Read the model definition and answer for the solid it produces. Units are mm, in the model's axes. A direction names the side the tool comes from. Coordinates: 2 decimals unless noted, no trailing zeros. Write each loop counter-clockwise with the first axis right and the second up, starting at its lowest first coordinate (ties: lowest second). Pieces come first, ordered by that corner, then holes. Notation, with made-up numbers: (50.5, 24.25) -> (62.5, 24.25) arc R16 cw to (62.5, 30.25) -> close; hole circle Ø6 at (63.5, 89). An arc over 180 degrees is marked (long way). Return JSON: item names as keys, results as strings.
Autodesk Inventor part; units mm, degrees
ref_plane "YZ Plane" through (0, 0, 0) normal (1, 0, 0) x (0, 1, 0)
ref_plane "XZ Plane" through (0, 0, 0) normal (0, 1, 0) x (-1, 0, 0)
ref_plane "XY Plane" through (0, 0, 0) normal (0, 0, 1) x (1, 0, 0)
sketch "스케치1" plane through (0, 0, 0) normal (0, 1, 0) x (-1, 0, 0)
  line L0 (24.089, 25.4241) -> (-27.911, 25.4241)
  line L1 (-27.911, 25.4241) -> (-27.911, -26.5759)
  line L2 (-27.911, -26.5759) -> (24.089, -26.5759)
  line L3 (24.089, -26.5759) -> (24.089, 25.4241)
  point P0 (0, 0)
  dimension "d0" = 52
  dimension "d1" = 52
extrude "돌출2" add sketch "스케치1" along normal blind 5
sketch "스케치2" plane through (0, 0, 0) normal (0, -1, 0) x (1, 0, 0)
  line L0 (27.911, 25.4241) -> (27.911, -26.5759)
  line L1 (-24.089, 25.4241) -> (27.911, 25.4241)
  line L2 (-24.089, -26.5759) -> (-24.089, 25.4241)
  line L3 (27.911, -26.5759) -> (-24.089, -26.5759)
  line L4 (-24.089, 25.4241) -> (-19.089, 25.4241)
  line L5 (-19.089, 25.4241) -> (-19.089, -26.5759)
  line L6 (-19.089, -26.5759) -> (-24.089, -26.5759)
  line L7 (-24.089, -26.5759) -> (-24.089, 25.4241)
  line L8 (27.911, 25.4241) -> (22.911, 25.4241)
  line L9 (22.911, 25.4241) -> (22.911, -26.5759)
  line L10 (22.911, -26.5759) -> (27.911, -26.5759)
  line L11 (27.911, -26.5759) -> (27.911, 25.4241)
  point P0 (0, 0)
  dimension "d8" = 5
  dimension "d9" = 5
extrude "돌출3" add sketch "스케치2" along normal blind 42 contours L0 L3 L9 L1 | L5 L3 L2 L1
sketch "스케치4" plane through (0, 5, 0) normal (0, 1, 0) x (1, 0, 0)
  line L0 (27.911, -25.4241) -> (27.911, 26.5759)
  line L1 (27.911, 26.5759) -> (-24.089, 26.5759)
  line L2 (-24.089, 26.5759) -> (-24.089, -25.4241)
  line L3 (-24.089, -25.4241) -> (27.911, -25.4241)
  line L4 (27.911, 26.5759) -> (38.911, 26.5759)
  line L5 (38.911, 26.5759) -> (38.911, -25.4241)
  line L6 (38.911, -25.4241) -> (27.911, -25.4241)
  line L7 (27.911, -25.4241) -> (27.911, 26.5759)
  line L8 (-24.089, 26.5759) -> (-36.089, 26.5759)
  line L9 (-36.089, 26.5759) -> (-36.089, -25.4241)
  line L10 (-36.089, -25.4241) -> (-24.089, -25.4241)
  line L11 (-24.089, -25.4241) -> (-24.089, 26.5759)
  line L12 (-24.089, 26.5759) -> (27.911, 26.5759)
  line L13 (27.911, 26.5759) -> (27.911, -25.4241)
  line L14 (27.911, -25.4241) -> (-24.089, -25.4241)
  line L15 (-24.089, -25.4241) -> (-24.089, 26.5759)
  line L16 (-24.089, -15.4219) -> (-4.089, -25.4241)
  point P0 (0, 0)
  point P1 (-24.089, -25.4241)
  dimension "d12" = 11
  dimension "d13" = 12
  dimension "d32" = 0
  dimension "d33" = 52
  dimension "d34" = 52
  dimension "d35" = 0
  dimension "d36" = 52
  dimension "d37" = 52
  dimension "d38" = 26.57
  dimension "d39" = 20
sketch "스케치8" plane through (27.911, -42, 25.4241) normal (1, 0, 0) x (0, 0, -1)
  line L0 (52, 0) -> (52, 47)
  line L1 (0, 47) -> (52, 47)
  line L2 (0, 47) -> (0, 0)
  line L3 (52, 0) -> (0, 0)
  circle A0 centre (26, 16.074) radius 4.5
  point P0 (25.4241, 42)
  point P1 (26, 0)
  dimension "d26" = 9
  dimension "d27" = 16.074
extrude "돌출8" cut sketch "스케치8" along normal mid plane 150 contours A0
properties part number "new_camera_case_front"
1. For a pull along X with two mould halves and no side action, classify faces 1 (the face through (-24.089, -19, -1)), 2 (the face through (-22, -42, 0)), 3 (the face through (22.911, -21, 0)) as +X half, -X half, draft (parallel to the pull), parting line (faces both ways), or undercut.
Taken from the geometry:
{"face 1": "-X half", "face 2": "draft", "face 3": "undercut"}
2. A flat-ended cylindrical pin translates along its axis: pin 1 Ø7 at (y, z) = (-25.93, -0.58) entering from -X. Find the tip coordinate at first contact, or state that the pin passes through.
Taken from the geometry:
{"pin 1": "passes through"}
3. The part is cut by section A-A (y = -38). Determine the outline of the cut face in (x, z).
Taken from the geometry:
{"outline": "(-24.09, -26.58) -> (-19.09, -26.58) -> (-19.09, 25.42) -> (-24.09, 25.42) -> close; (22.91, -26.58) -> (27.91, -26.58) -> (27.91, 25.42) -> (22.91, 25.42) -> close"}
4. The part is cut by section D-D (x = -17). Determine the outline of the cut face in (y, z).
Taken from the geometry:
{"outline": "(0, -26.58) -> (5, -26.58) -> (5, 25.42) -> (0, 25.42) -> close"}
5. The part is cut by section C-C (z = 22). Determine the outline of the cut face in (x, y).
Taken from the geometry:
{"outline": "(-24.09, -42) -> (-19.09, -42) -> (-19.09, 0) -> (22.91, 0) -> (22.91, -42) -> (27.91, -42) -> (27.91, 5) -> (-24.09, 5) -> close"}
6. A tool of negligible diameter and unlimited length cuts with its end or side. For faces 4 (the face through (-19.089, -21, 0)), 5 (the face through (-21.55, -29.92, -2.65)), from which of +Z, -Z, +X, -X, +Y, -Y can it reach the whole face along a straight path? Write none if from no direction.
Taken from the geometry:
{"face 4": "+Z, -Z, -Y", "face 5": "+X, -X"}
7. Consider L1, parallel to X at y = -32, z = -19; L2, parallel to Y at x = 14, z = -22. Determine where each line is inside the solid, lowest interval first.
Taken from the geometry:
{"L1": "x = -24.09 to -19.09, 22.91 to 27.91", "L2": "y = 0 to 5"}
8. The part is cut by section B-B (y = -28). Determine the outline of the cut face in (x, z), then the cut area to 3 significant figures.
Taken from the geometry:
{"outline": "(-24.09, -26.58) -> (-19.09, -26.58) -> (-19.09, -4.57) -> (-24.09, -4.57) -> close; (-24.09, 3.42) -> (-19.09, 3.42) -> (-19.09, 25.42) -> (-24.09, 25.42) -> close; (22.91, -26.58) -> (27.91, -26.58) -> (27.91, -4.57) -> (22.91, -4.57) -> close; (22.91, 3.42) -> (27.91, 3.42) -> (27.91, 25.42) -> (22.91, 25.42) -> close", "area": "440 mm2"}
